Geometry: final body of the model. Coordinates: model frame, mm. Face numbers are marked on the shaded views. A direction names the side the tool comes from. Round coordinates to 2 decimals unless told otherwise and drop trailing zeros. Order: outer loops, then holes, each group sorted by start corner. A loop starts at its lowest first (then second) coordinate and runs counter-clockwise, first axis right, second up. Notation, with made-up numbers: (36.25, 68.5) -> (46.25, 68.5) arc R11 ccw to (46.25, 86.5) -> close; hole circle Ø11 at (50.25, 8). An arc over 180 degrees is marked (long way). Put each result on its own line as item: value.
```python
from build123d import *

# Parameters (mm, degrees)
RESSALTO_EXTRUS_O1_DEPTH   = 10
RESSALTO_EXTRUS_O1_2_DEPTH = 10
ESBO_O2_W                  = 9
ESBO_O2_H                  = 70
RESSALTO_EXTRUS_O2_DEPTH   = 2
ESBO_O3_W                  = 3
ESBO_O3_H                  = 52
CORTE_EXTRUS_O1_DEPTH      = 3


with BuildPart() as part:
    # Esbo_o1 → Ressalto-extrus_o1 (new body)
    with BuildSketch(Plane(origin=(0, 0, 0), x_dir=(1, 0, 0), z_dir=(0, 1, 0))):
        Polygon((0.5, -30), (0.5, -35), (4.5, -35), (4.5, -26), (-4.5, -26), (-4.5, -30), align=None)
    extrude(amount=RESSALTO_EXTRUS_O1_DEPTH)



with BuildPart() as body_2:
    # Esbo_o1 → Ressalto-extrus_o1 2 (new body)
    with BuildSketch(Plane(origin=(0, 0, 0), x_dir=(1, 0, 0), z_dir=(0, 1, 0))):
        Polygon((-4.5, 30), (-4.5, 26), (4.5, 26), (4.5, 35), (0.5, 35), (0.5, 30), align=None)
    extrude(amount=RESSALTO_EXTRUS_O1_2_DEPTH)


with BuildPart() as part_1:
    add(part.part)

    add(body_2.part)  # Ressalto-extrus_o2 merges body 2
    # Esbo_o2 → Ressalto-extrus_o2 (add)
    with BuildSketch(Plane(origin=(0, 0, 0), x_dir=(1, 0, 0), z_dir=(0, 1, 0))):
        Rectangle(ESBO_O2_W, ESBO_O2_H)
    extrude(amount=RESSALTO_EXTRUS_O2_DEPTH)

    # Esbo_o3 → Corte-extrus_o1 (cut, through all)
    with BuildSketch(Plane(origin=(0, 2, 0), x_dir=(1, 0, 0), z_dir=(0, 1, 0))):
        with Locations((3, 0)):
            Rectangle(ESBO_O3_W, ESBO_O3_H)
    extrude(amount=-CORTE_EXTRUS_O1_DEPTH, mode=Mode.SUBTRACT)


solid = part_1.part
```
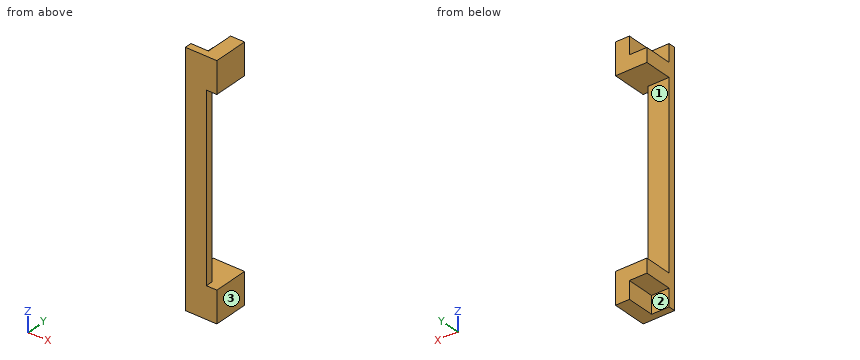
1. Cut plane A-A on x = 2.5. Return loops of the section in (y, z).
Ans:
outline: (0, -35) -> (10, -35) -> (10, -26) -> (0, -26) -> close; (0, 26) -> (10, 26) -> (10, 35) -> (0, 35) -> close
2. Cut plane D-D on z = -15.5. Return loops of the section in (x, y), and give its area (3 significant figures).
Ans:
outline: (-4.5, 0) -> (1.5, 0) -> (1.5, 2) -> (-4.5, 2) -> close
area: 12.0 mm²
3. Set-up query: the marked faces 1, 2 and 3. Return all of +Z, -Z, +X, -X, +Y, -Y with unobstructed straight access to the full face (end or side cutting, diameter ignored); none if empty.
Ans:
face 1: +X, -X, +Y
face 2: -Z, -X, +Y
face 3: +Z, -Z, +X, +Y, -Y
4. Material intervals for probe 1 along Z at (x, y) = (-1.5, 3.25); probe 2 along Z at (x, y) = (2.25, 6.5); probe 3 along Y at (x, z) = (0.5, -24), sorted ascending.
Ans:
probe 1: -30 to -26, 26 to 30
probe 2: -35 to -26, 26 to 35
probe 3: 0 to 2
5. Contact query for flat-ended pins moving along their axis: P1, Ø1.5, axis at x = -2.5, z = 18.5, coming from the +Y side; P2, Ø1.5, axis at y = 7.5, z = -33, coming from the -X side; P3, Ø2.5, axis at x = -1, y = 4, coming from the -Z side. Output: stop coordinate, or through.
Ans:
P1: y = 2
P2: x = 0.5
P3: z = -30
6. Cut plane B-B on y = 3.25. Return loops of the section in (x, z), and give its area (3 significant figures).
Ans:
outline: (-4.5, -30) -> (0.5, -30) -> (0.5, -35) -> (4.5, -35) -> (4.5, -26) -> (-4.5, -26) -> close; (-4.5, 26) -> (4.5, 26) -> (4.5, 35) -> (0.5, 35) -> (0.5, 30) -> (-4.5, 30) -> close
area: 112 mm²
7. Cut plane C-C on x = -1.75. Return loops of the section in (y, z).
Ans:
outline: (0, -35) -> (2, -35) -> (2, -30) -> (10, -30) -> (10, -26) -> (2, -26) -> (2, 26) -> (10, 26) -> (10, 30) -> (2, 30) -> (2, 35) -> (0, 35) -> close
